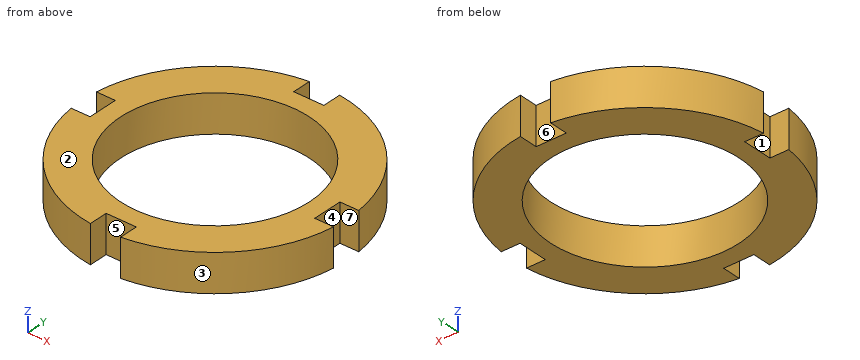
```python
from build123d import *

# Parameters (mm, degrees)
SKETCH1_R           = 12.5
BOSS_EXTRUDE1_DEPTH = 5


with BuildPart() as part:
    # Sketch1 → Boss-Extrude1 (new body)
    with BuildSketch(Plane.XY):
        with BuildLine():
            Line((17.385338651, 2), (14.885338651, 2))
            Line((14.885338651, 2), (14.885338651, -2))
            Line((14.885338651, -2), (17.385338651, -2))
            ThreePointArc((17.385338651, -2), (12.374368671, -12.374368671), (2, -17.385338651))
            Line((2, -17.385338651), (2, -14.885338651))
            Line((2, -14.885338651), (-2, -14.885338651))
            Line((-2, -14.885338651), (-2, -17.385338651))
            ThreePointArc((-2, -17.385338651), (-12.374368671, -12.374368671), (-17.385338651, -2))
            Line((-17.385338651, -2), (-14.885338651, -2))
            Line((-14.885338651, -2), (-14.885338651, 2))
            Line((-14.885338651, 2), (-17.385338651, 2))
            ThreePointArc((-17.385338651, 2), (-12.374368671, 12.374368671), (-2, 17.385338651))
            Line((-2, 17.385338651), (-2, 14.885338651))
            Line((-2, 14.885338651), (2, 14.885338651))
            Line((2, 14.885338651), (2, 17.385338651))
            ThreePointArc((2, 17.385338651), (12.374368671, 12.374368671), (17.385338651, 2))
        make_face()
        Circle(SKETCH1_R, mode=Mode.SUBTRACT)
    extrude(amount=BOSS_EXTRUDE1_DEPTH)


solid = part.part
```
For this review, take the finished solid that the model builds, in its own axes (mm). Face numbers are marked on the shaded views. A direction names the side the tool comes from. Round coordinates to 2 decimals unless told otherwise and drop trailing zeros. Write each loop counter-clockwise with the first axis right and the second up, starting at its lowest first coordinate (ties: lowest second). Pieces come first, ordered by that corner, then holes. Notation, with made-up numbers: (32, 27) - (59, 27) arc R32 cw to (59, 54) - close; hole circle Ø10 at (88.25, 67.5). An arc over 180 degrees is marked (long way). Write each question's results on one line, items separated by ' | '.
Item 1: For pin 1 (1.3 mm diameter, centred on x = -16, z = 1.5, fed in from +Y); pin 2 (2 mm diameter, centred on y = -16, z = 3, fed in from -X); pin 3 (3 mm diameter, centred on y = 1, z = 3, fed in from -X), all flat-tipped, find the tip position at first contact; note any pin that passes through.
Calculated:
pin 1: stops at y = 8.4 | pin 2: stops at x = -9.01 | pin 3: stops at x = -17.39
Item 2: Take a section at D-D on x = 14. State the section outline as (y, z) points, then the cut area to 3 significant figures.
Calculated:
outline: (-10.5, 0) - (10.5, 0) - (10.5, 5) - (-10.5, 5) - close | area: 105 mm^2
Item 3: Take a section at A-A on z = 1.1. State the section outline as (x, y) points.
Calculated:
outline: (-17.39, -2) arc R17.5 ccw to (-2, -17.39) - (-2, -14.89) - (2, -14.89) - (2, -17.39) arc R17.5 ccw to (17.39, -2) - (14.89, -2) - (14.89, 2) - (17.39, 2) arc R17.5 ccw to (2, 17.39) - (2, 14.89) - (-2, 14.89) - (-2, 17.39) arc R17.5 ccw to (-17.39, 2) - (-14.89, 2) - (-14.89, -2) - close; hole circle Ø25 at (0, 0)
Item 4: To check wall thickness, follow line 1 along Y through (x, z) = (0, 2.5); line 2 along X through (y, z) = (-5, 1.8); line 3 along X through (y, z) = (9, 3.25). State the ranges of each line that lie inside material, in increasing order. Write a range as from..to.
Calculated:
line 1: y = -14.89..-12.5, 12.5..14.89 | line 2: x = -16.77..-11.46, 11.46..16.77 | line 3: x = -15.01..-8.67, 8.67..15.01
Item 5: Draft analysis for pull direction Y (two halves, no side actions). For the marked faces 1, 2, 3 and 4, state which applies: pulls with the +Y half, pulls with the -Y half, needs draft (parallel to the pull), parting line crosses it, or undercut.
Calculated:
face 1: undercut | face 2: needs draft | face 3: pulls with the -Y half | face 4: undercut
Item 6: For the marked faces 5, 6 and 7, list the 3-axis set-ups (+Z, -Z, +X, -X, +Y, -Y) from which the entire face can be reached by the end or side of a thin tool; tool diameter is ignored.
Calculated:
face 5: +Z, -Z, -Y | face 6: +Z, -Z, +Y | face 7: +Z, -Z, +X
Item 7: Take a section at B-B on y = 0. State the section outline as (x, z) points, then the cut area to 3 significant figures.
Calculated:
outline: (-14.89, 0) - (-12.5, 0) - (-12.5, 5) - (-14.89, 5) - close; (12.5, 0) - (14.89, 0) - (14.89, 5) - (12.5, 5) - close | area: 23.9 mm^2
